from build123d import *

# Parameters (mm, degrees)
F0_R     = 4.25
F1_DEPTH = 5
F2_R     = 2.5
F3_DEPTH = 25
F4_R     = 2.5
F4_R_2   = 2.1
F5_DEPTH = 22
F7_DEPTH = 2.5
F8_SIZE  = 0.4


with BuildPart() as f1:
    # F0 (on Front) → F1 (new body)
    with BuildSketch(Plane.XZ):
        Circle(F0_R)
    extrude(amount=F1_DEPTH)

    # F2 (on face) → F3 (join)
    with BuildSketch(Plane(origin=(0, 0, 0), x_dir=(-1, 0, 0), z_dir=(0, 1, 0))):
        Circle(F2_R)
    extrude(amount=F3_DEPTH)

    # F4 (on face) → F5 (cut)
    with BuildSketch(Plane(origin=(0, 25, 0), x_dir=(-1, 0, 0), z_dir=(0, 1, 0))):
        Circle(F4_R)
        Circle(F4_R_2, mode=Mode.SUBTRACT)
    extrude(amount=-F5_DEPTH, mode=Mode.SUBTRACT)

    # F6 (on face) → F7 (cut)
    with BuildSketch(Plane.XZ.offset(5)):
        Polygon((0, -2.309401), (2, -1.154701), (2, 1.154701), (0, 2.309401), (-2, 1.154701), (-2, -1.154701), align=None)
    extrude(amount=-F7_DEPTH, mode=Mode.SUBTRACT)

    # F8
    f8_edges = [f1.edges().sort_by_distance(p)[0] for p in [
        (-4.25, -5, 0),
    ]]
    chamfer(f8_edges, length=F8_SIZE)


solid = f1.part
Geometry: final body of the model. Coordinates: model frame, mm. A direction names the side the tool comes from. Give positions to 0.01 mm unless a question says otherwise; leave off trailing zeros. Write each loop counter-clockwise with the first axis right and the second up, starting at its lowest first coordinate (ties: lowest second). Pieces come first, ordered by that corner, then holes. Notation, with made-up numbers: (13.5, 72) - (60.5, 72) arc R18 cw to (60.5, 105) - close; hole circle Ø1 at (12.5, 82). An arc over 180 degrees is marked (long way). Return JSON: item names as keys, results as strings. Group by question number.
1) Section A-A on z = 0. Return the cut outline in (x, y), plus the area to 3 significant figures.
2) Section B-B on y = -1.75. Return the cut outline in (x, z), plus the area to 3 significant figures.
3) Section C-C on y = 6.5. Return the cut outline in (x, z), plus the area to 3 significant figures.
4) Mould query, pull axis X, two halves, no side actions, for faces 4 (the cylindrical face through (2.285, -2.268, 3.584)), 5 (the flat face through (0, 25, 0)), 6 (the flat face through (-0.99, -3.77, 1.74)). Classes: released by +X, released by -X, zero draft, split by the parting line, or undercut.
5) Set-up query: faces 1 (the flat face through (2, -5, -2)), 2 (the flat face through (0, -2.5, 0)), 3 (the flat face through (2, 0, -2)). Return all of +Z, -Z, +X, -X, +Y, -Y with unobstructed straight access to the full face (end or side cutting, diameter ignored); none if empty.
6) Line query: line 1 (Z direction, x = 0, y = 10.5); line 2 (Z direction, x = 1.75, y = 3.25); line 3 (Y direction, x = -2.5, z = -0.5). Output: solid intervals per line, ascending.
7) First-contact query: P1, Ø4, axis at x = 1.5, y = 12, coming from the -Z side; P2, Ø2, axis at x = 1.5, y = 21, coming from the -Z side; P3, Ø1, axis at y = 4, z = -1, coming from the -X side. Flat tips, straight axial feed; report the tip coordinate or a pass-through.
Filled in:
{
 "1": {"outline": "(-4.25, -4.6) - (-3.85, -5) - (-2, -5) - (-2, -2.5) - (2, -2.5) - (2, -5) - (3.85, -5) - (4.25, -4.6) - (4.25, 0) - (2.5, 0) - (2.5, 3) - (2.1, 3) - (2.1, 25) - (-2.1, 25) - (-2.1, 3) - (-2.5, 3) - (-2.5, 0) - (-4.25, 0) - close", "area": "140 mm^2"},
 "2": {"outline": "circle Ø8.5 at (0, 0)", "area": "56.7 mm^2"},
 "3": {"outline": "circle Ø4.2 at (0, 0)", "area": "13.9 mm^2"},
 "4": {"face 4": "split by the parting line", "face 5": "zero draft", "face 6": "undercut"},
 "5": {"face 1": "+Z, -Z, +X, -X, -Y", "face 2": "-Y", "face 3": "+Y"},
 "6": {"line 1": "z = -2.1 to 2.1", "line 2": "z = -1.16 to 1.16", "line 3": "y = -5 to 0"},
 "7": {"P1": "stops at z = -2.1", "P2": "stops at z = -2.04", "P3": "stops at x = -2.04"}
}
